Could you check a few things on this model? Use its own coordinates, in mm. A direction names the side the tool comes from. Give positions to 0.01 mm unless a question says otherwise; leave off trailing zeros. Loops run counter-clockwise (first coordinate to the right, second up) from the corner with the lowest first, then second, coordinate; pieces in that order, holes last. Notation, with made-up numbers: (79, 29.5) -> (136, 29.5) arc R19 ccw to (136, 36.5) -> close; hole circle Ø3 at (47, 12.25). An arc over 180 degrees is marked (long way). Put each result on its own line as item: value.
```python
from build123d import *

# Parameters (mm, degrees)
F0_W     = 100
F0_H     = 100
F2_DEPTH = 10
F3_R     = 5.08
F4_DEPTH = 61.976


# Not quite as in the source:
# - a feature of the source that left no trace in its solid (it failed there, or was rolled back) is left out


with BuildPart() as f2:
    # F0 (on Top) → F2 (new body)
    with BuildSketch(Plane.XY):
        Rectangle(F0_W, F0_H)
    extrude(amount=F2_DEPTH)

    # F3
    f3_edges = [f2.edges().sort_by_distance(p)[0] for p in [
        (0, 50, 10),
        (-50, 0, 10),
        (0, -50, 10),
        (50, 0, 10),
    ]]
    fillet(f3_edges, radius=F3_R)

    # F1 (on face) → F4 (cut)
    with BuildSketch(Plane.XY):
        Polygon((-11.7515370065, 14.8558261646), (-18.8142469277, 2.1950639145), (-14.8558261646, -11.7515370065), (-2.1950639145, -18.8142469277), (11.7515370065, -14.8558261646), (18.8142469277, -2.1950639145), (14.8558261646, 11.7515370065), (2.1950639145, 18.8142469277), align=None)
    extrude(amount=F4_DEPTH, mode=Mode.SUBTRACT)


solid = f2.part
```
1. For faces 1 (the face through (0.7, 48.551, 8.472)), 2 (the face through (-16.863, -4.681, 4.93)), which set-ups out of +Z, -Z, +X, -X, +Y, -Y let a thin tool reach every point of the face, with its end or its side?
Recorded:
face 1: +Z, +X, -X, +Y
face 2: +Z, -Z
2. I'm going to push flat-ended pins straight in: pin 1 (3 mm diameter, centred on x = -35.5, z = 8, fed in from +Y); pin 2 (1.5 mm diameter, centred on y = 19, z = 8, fed in from -X). Where does each tip first touch, or does it pass through?
Recorded:
pin 1: stops at y = 49.75
pin 2: stops at x = -49.43
3. I need wall thicknesses on line 1 (X direction, y = -1.5, z = 2.75); line 2 (X direction, y = 4.5, z = 7.5); line 3 (Y direction, x = -7, z = 0.75). Which ranges of each line are inside material? Lowest first, please.
Recorded:
line 1: x = -50 to -17.77, 18.62 to 50
line 2: x = -49.3 to -17.53, 16.91 to 49.3
line 3: y = -50 to -16.13, 16.2 to 50
4. If we section it at A-A (z = 3): List the corners of the cut face in (x, y) for me, then the cut area to 3 significant figures.
Recorded:
outline: (-50, -50) -> (50, -50) -> (50, 50) -> (-50, 50) -> close; hole (-18.81, 2.2) -> (-14.86, -11.75) -> (-2.2, -18.81) -> (11.75, -14.86) -> (18.81, -2.2) -> (14.86, 11.75) -> (2.2, 18.81) -> (-11.75, 14.86) -> close
area: 8,990 mm^2
5. Thinking about a two-plate mould opening in Y: for faces 3 (the face through (8.614, 15.233, 4.93)), 4 (the face through (-48.551, 0.7, 8.472)), 5 (the face through (-1, 50, 2)), 6 (the face through (16.863, 4.681, 4.93)), which applies, pulls with the +Y half, pulls with the -Y half, needs draft (parallel to the pull), parting line crosses it, or undercut?
Recorded:
face 3: undercut
face 4: needs draft
face 5: pulls with the +Y half
face 6: undercut
